from build123d import *

# Parameters (mm, degrees)
F0_R     = 38.1
F1_DEPTH = 12.7
F2_R     = 31.75
F3_DEPTH = 11.43
F4_R     = 5.08


with BuildPart() as f1:
    # F0 (on Front) → F1 (new body)
    with BuildSketch(Plane.XZ):
        Circle(F0_R)
    extrude(amount=F1_DEPTH)

    # F2 (on face) → F3 (cut)
    with BuildSketch(Plane(origin=(0, 0, 0), x_dir=(-1, 0, 0), z_dir=(0, 1, 0))):
        Circle(F2_R)
    extrude(amount=-F3_DEPTH, mode=Mode.SUBTRACT)

    # F4
    f4_edges = [f1.edges().sort_by_distance(p)[0] for p in [
        (38.1, -6.35, 0),
        (-38.1, 0, 0),
        (-38.1, -12.7, 0),
    ]]
    fillet(f4_edges, radius=F4_R)


solid = f1.part
Verification items for the finished model (mm, model axes). A direction names the side the tool comes from. Give positions to 0.01 mm unless a question says otherwise; leave off trailing zeros. Loops run counter-clockwise (first coordinate to the right, second up) from the corner with the lowest first, then second, coordinate; pieces in that order, holes last. Notation, with made-up numbers: (62, -3.5) - (84, -3.5) arc R5 cw to (84, 4.5) - close; hole circle Ø4 at (54.5, -22). An arc over 180 degrees is marked (long way). Write item = value, one per line. Start each with the question number.
Q1. Cross-section at B-B, the plane z = 0. Enter the section's corners in (x, y).
Q2. Cross-section at D-D, the plane y = -1.5. Enter the section's corners in (x, z).
Q3. Cross-section at A-A, the plane x = 0. Enter the section's corners in (y, z).
Q4. Cross-section at C-C, the plane y = -6.75. Enter the section's corners in (x, z), and give its area (3 significant figures).
Q5. Tool access check on faces 1 (the face through (6.883, -5.635, -30.995)), 2 (the face through (0, -12.7, 0)). Record the directions out of +Z, -Z, +X, -X, +Y, -Y that give a thin tool (end or side, any length) a straight path to the whole face; none if there is none.
Q6. Mould release check, pull along Z, two halves, no side actions. Record for faces 3 (the face through (-30.235, -6.332, -23.183)), 4 (the face through (-17, 0, 27)), 5 (the face through (0, -11.43, 0)): released by +Z, released by -Z, zero draft, split by the parting line, or undercut.
Q7. Depth check by flat-ended pin: P1, Ø4, axis at y = -9, z = -16.5, coming from the +X side; P2, Ø3, axis at x = 10, z = -10.5, coming from the +Y side; P3, Ø6, axis at x = -26, y = -2, coming from the +Z side. Enter the tip coordinate at first touch or a pass-through.
Q8. Thickness scan on line 1 (Z direction, x = 0, y = -7.75); line 2 (X direction, y = -4.75, z = -1); line 3 (Y direction, x = -15, z = -5.5). Record the ranges inside material, lowest first.
Answer key:
q1.outline = (-38.1, -7.62) arc R5.08 ccw to (-33.02, -12.7) - (33.02, -12.7) arc R5.08 ccw to (38.1, -7.62) - (38.1, -5.08) arc R5.08 ccw to (33.02, 0) - (31.75, 0) - (31.75, -11.43) - (-31.75, -11.43) - (-31.75, 0) - (-33.02, 0) arc R5.08 ccw to (-38.1, -5.08) - close
q2.outline = circle Ø73.25 at (0, 0); hole circle Ø63.5 at (0, 0)
q3.outline = (-12.7, -33.02) arc R5.08 ccw to (-7.62, -38.1) - (-5.08, -38.1) arc R5.08 ccw to (0, -33.02) - (0, -31.75) - (-11.43, -31.75) - (-11.43, 31.75) - (0, 31.75) - (0, 33.02) arc R5.08 ccw to (-5.08, 38.1) - (-7.62, 38.1) arc R5.08 ccw to (-12.7, 33.02) - close
q4.outline = circle Ø76.2 at (0, 0); hole circle Ø63.5 at (0, 0)
q4.area = 1,390 mm^2
q5.face_1 = +Y
q5.face_2 = +Z, -Z, +X, -X, -Y
q6.face_3 = split by the parting line
q6.face_4 = zero draft
q6.face_5 = undercut
q7.P1 = 35.13
q7.P2 = -11.43
q7.P3 = 29.75
q8.line_1 = -38.1 to -31.75, 31.75 to 38.1
q8.line_2 = -38.08 to -31.73, 31.73 to 38.08
q8.line_3 = -12.7 to -11.43
